For this review, take the finished solid that the model builds, in its own axes (mm). Face numbers are marked on the shaded views. Round coordinates to 2 decimals unless told otherwise and drop trailing zeros. Order: outer loops, then holes, each group sorted by start corner. A loop starts at its lowest first (then second) coordinate and runs counter-clockwise, first axis right, second up.
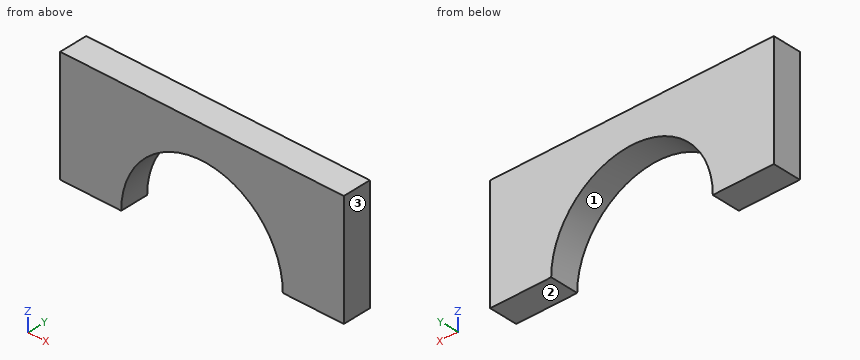
```python
from build123d import *

# Parameters (mm, degrees)
EXTRUDE_1_DEPTH = 20


with BuildPart() as part:
    # Эскиз1 → Бобышка-Вытянуть1 (new body)
    with BuildSketch(Plane(origin=(0, 0, 0), x_dir=(1, 0, 0), z_dir=(0, 1, 0))):
        with BuildLine():
            Line((-100, 0), (100, 0))
            Line((100, 0), (100, 80))
            Line((100, 80), (57, 80))
            ThreePointArc((57, 80), (0, 23), (-57, 80))
            Line((-57, 80), (-100, 80))
            Line((-100, 80), (-100, 0))
        make_face()
    extrude(amount=EXTRUDE_1_DEPTH)


solid = part.part
```
Q1. Take a section at D-D, the plane z = -66. State the section outline as (x, y) points, plus the area to 3 significant figures.
Q2. Take a section at A-A, the plane z = -53.5. State the section outline as (x, y) points, plus the area to 3 significant figures.
Q3. Take a section at B-B, the plane y = 5.5. State the section outline as (x, z) points, plus the area to 3 significant figures.
Q4. Mouldability with a two-part tool opening along X and no side actions: class the marked faces 1, 2 and 3 as +X half, -X half, draft (parallel to the pull), parting line (faces both ways), or undercut.
Q5. Take a section at C-C, the plane x = 0. State the section outline as (y, z) points.
Q6. Wall thickness on line 1 (X direction, y = 12.25, z = -75); line 2 (X direction, y = 11.5, z = -28); line 3 (Z direction, x = 17, y = 16.25): over which ranges is each line inside the solid? List them lowest first.
Working result:
1. outline: (-100, 0) - (-55.25, 0) - (-55.25, 20) - (-100, 20) - close; (55.25, 0) - (100, 0) - (100, 20) - (55.25, 20) - close
1. area: 1,790 mm2
2. outline: (-100, 0) - (-50.47, 0) - (-50.47, 20) - (-100, 20) - close; (50.47, 0) - (100, 0) - (100, 20) - (50.47, 20) - close
2. area: 1,980 mm2
3. outline: (-100, -80) - (-57, -80) arc R57 cw to (57, -80) - (100, -80) - (100, 0) - (-100, 0) - close
3. area: 10,900 mm2
4. face 1: undercut
4. face 2: draft
4. face 3: +X half
5. outline: (0, -23) - (20, -23) - (20, 0) - (0, 0) - close
6. line 1: x = -100 to -56.78, 56.78 to 100
6. line 2: x = -100 to -23.35, 23.35 to 100
6. line 3: z = -25.59 to 0
